```python
from build123d import *

# Parameters (mm, degrees)
SKETCH_R        = 42.5
PAD_DEPTH       = 2
SKETCH001_R     = 40
PAD001_DEPTH    = 10
SKETCH002_R     = 7.5
POCKET_DEPTH    = 6
SKETCH003_W     = 7.6
SKETCH003_H     = 27.2
POCKET001_DEPTH = 6
FILLET_R        = 6
FILLET001_R     = 3.7999
SKETCH004_R     = 1.55
POCKET002_DEPTH = 6
SKETCH005_R     = 3
POCKET003_DEPTH = 3
SKETCH006_R     = 1.55
POCKET004_DEPTH = 12


with BuildPart() as part:
    # Sketch → Pad (new body)
    with BuildSketch(Plane.XY):
        Circle(SKETCH_R)
    extrude(amount=PAD_DEPTH)

    # Sketch001 (on Face3 of Pad) → Pad001 (join)
    with BuildSketch(Plane.XY.offset(2)):
        Circle(SKETCH001_R)
    extrude(amount=PAD001_DEPTH)

    # Sketch002 (on Face5 of Pad001) → Pocket (cut)
    with BuildSketch(Plane.XY.offset(12)):
        Circle(SKETCH002_R)
    extrude(amount=-POCKET_DEPTH, mode=Mode.SUBTRACT)

    # Sketch003 (on Face5 of Pocket) → Pocket001 (cut)
    with BuildSketch(Plane.XY.offset(12)):
        with Locations((0, 13.6)):
            Rectangle(SKETCH003_W, SKETCH003_H)
    extrude(amount=-POCKET001_DEPTH, mode=Mode.SUBTRACT)

    # Fillet
    fillet_edges = [part.edges().sort_by_distance(p)[0] for p in [
        (-3.8, 6.466065, 9),
        (3.8, 6.466065, 9),
    ]]
    fillet(fillet_edges, radius=FILLET_R)

    # Fillet001
    fillet001_edges = [part.edges().sort_by_distance(p)[0] for p in [
        (3.8, 27.2, 9),
        (-3.8, 27.2, 9),
    ]]
    fillet(fillet001_edges, radius=FILLET001_R)

    # Sketch004 (on Face12 of Fillet001) → Pocket002 (cut)
    with BuildSketch(Plane.XY.offset(6)):
        with Locations((0, 23.5)):
            Circle(SKETCH004_R)
    extrude(amount=-POCKET002_DEPTH, mode=Mode.SUBTRACT)

    # Sketch005 (on Face13 of Pocket002) → Pocket003 (cut)
    with BuildSketch(Plane.XY.offset(6)):
        Circle(SKETCH005_R)
    extrude(amount=-POCKET003_DEPTH, mode=Mode.SUBTRACT)

    # Sketch006 (on Face1 of Pocket003) → Pocket004 (cut)
    with BuildSketch(Plane.XY.offset(12)):
        with Locations((-15, 5)):
            Circle(SKETCH006_R)
        with Locations((15, 5)):
            Circle(SKETCH006_R)
        with Locations((15, -5)):
            Circle(SKETCH006_R)
        with Locations((-15, -5)):
            Circle(SKETCH006_R)
    extrude(amount=-POCKET004_DEPTH, mode=Mode.SUBTRACT)


solid = part.part
```
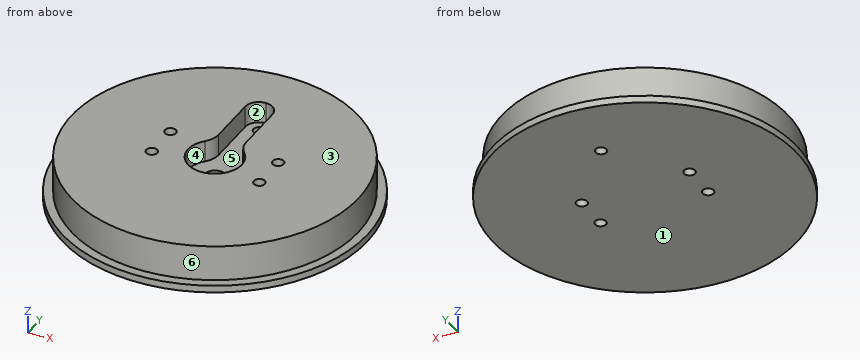
Geometry check sheet. Reference: the model listing, model coordinates, mm. Face numbers are marked on the shaded views. A direction names the side the tool comes from. Coordinates: 2 decimals unless noted, no trailing zeros. Order: outer loops, then holes, each group sorted by start corner. A loop starts at its lowest first (then second) coordinate and runs counter-clockwise, first axis right, second up. Notation, with made-up numbers: M 28,-15.5 L 64,-15.5 A15 cw 64,-6.5 Z; hole C 49.25,1 d2. An arc over 180 degrees is marked long. One line per question, with ' | ' between items. Start each with the question number.
Item 1: Cross-section at D-D on y = 13. Enter the section's corners in (x, z).
Item 2: Gauge pin test, flat ends, axial feed: pin 1 (2.5 mm diameter, centred on x = 15, y = 5, fed in from -Z); pin 2 (2 mm diameter, centred on x = 31, z = 7.5, fed in from -Y); pin 3 (6.5 mm diameter, centred on x = -0.5, y = 0.5, fed in from +Z); pin 4 (1.8 mm diameter, centred on y = 14, z = 8, fed in from -X). Record the tip position at first contact, or that the pin passes through.
Item 3: Draft check along X on the marked faces 3, 4, 5 and 6. Enter one of: pulls with the +X half, pulls with the -X half, needs draft (parallel to the pull), parting line crosses it, or undercut.
Item 4: Cross-section at C-C on x = 15. Enter the section's corners in (y, z), then the cut area to 3 significant figures.
Item 5: Cross-section at B-B on y = -5. Enter the section's corners in (x, z).
Item 6: Cross-section at A-A on z = 8.5. State how many separate pieces and enclosed holes the cut face has, then the cut area to 3 significant figures.
Item 7: Material ranges on L1, parallel to Y at x = -15, z = 9; L2, parallel to X at y = -6, z = 7.75; L3, parallel to Z at x = 30.5, y = 28, recorded low to high. Write a range as [from, to].
Item 8: Set-up check for the marked faces 1 and 2: record each of +Z, -Z, +X, -X, +Y, -Y from which the full face is reachable in a straight line by a thin tool's end or side.
Findings:
1) outline: M -40.46,0 L 40.46,0 L 40.46,2 L 37.83,2 L 37.83,12 L 3.8,12 L 3.8,6 L -3.8,6 L -3.8,12 L -37.83,12 L -37.83,2 L -40.46,2 Z
2) pin 1: passes through | pin 2: stops at y = -26.46 | pin 3: stops at z = 6 | pin 4: stops at x = -37.79
3) face 3: needs draft | face 4: undercut | face 5: undercut | face 6: parting line crosses it
4) outline: M -39.76,0 L -6.55,0 L -6.55,12 L -37.08,12 L -37.08,2 L -39.76,2 Z; M -3.45,0 L 3.45,0 L 3.45,12 L -3.45,12 Z; M 6.55,0 L 39.76,0 L 39.76,2 L 37.08,2 L 37.08,12 L 6.55,12 Z | area: 826 mm²
5) outline: M -42.2,0 L -16.55,0 L -16.55,12 L -39.69,12 L -39.69,2 L -42.2,2 Z; M -13.45,0 L 13.45,0 L 13.45,12 L 5.59,12 L 5.59,6 L -5.59,6 L -5.59,12 L -13.45,12 Z; M 16.55,0 L 42.2,0 L 42.2,2 L 39.69,2 L 39.69,12 L 16.55,12 Z
6) separate pieces: 1 | enclosed holes: 5 | area: 4,670 mm²
7) L1: y = [-37.08, -6.55], [-3.45, 3.45], [6.55, 37.08] | L2: x = [-39.55, -16.18], [-13.82, -4.5], [4.5, 13.82], [16.18, 39.55] | L3: z = [0, 2]
8) face 1: -Z, +X, -X, +Y, -Y | face 2: +Z
